The listing builds one solid part. Answer for the finished solid, in the listing's coordinates (mm). Face numbers are marked on the shaded views. A direction names the side the tool comes from. Give positions to 0.01 mm unless a question says otherwise; leave off trailing zeros. Order: outer loops, then holes, each group sorted by start corner. A loop starts at its lowest first (then second) coordinate and runs counter-clockwise, first axis right, second up. Notation, with made-up numbers: (-15, -8) - (4, -8) arc R27 cw to (4, 20) - close; hole circle Ø1 at (9, 21.5). An arc over 180 degrees is marked (long way). Answer as a JSON object with one key per item and string values. Group by question number.
Q1. The mould has two halves that part along X. Classify the marked faces 3, 4, 5 and 6: released by +X, released by -X, zero draft, split by the parting line, or undercut.
Q2. Given pin 1 (5 mm diameter, centred on y = 6.5, z = -6, fed in from +X); pin 2 (3.5 mm diameter, centred on x = -2, y = 10, fed in from -Z); pin 3 (1 mm diameter, centred on y = -6, z = -4, fed in from +X), each flat-ended and moving along its own axis, determine where each tip first touches the part or whether it passes through.
Q3. For the marked faces 1 and 2, determine the directions among +Z, -Z, +X, -X, +Y, -Y from which every point of the face is accessible in a straight line to the end or side of a thin tool.
Q4. A cutting plane is placed at D-D, the plane z = -6.75. Give the vertices of the cut face in (x, y), and give its area (3 significant figures).
Q5. A cutting plane is placed at B-B, the plane z = -1. Give the vertices of the cut face in (x, y), and give its area (3 significant figures).
Q6. A cutting plane is placed at A-A, the plane x = 0. Give the vertices of the cut face in (y, z), and give its area (3 significant figures).
Q7. A cutting plane is placed at C-C, the plane y = -17. Give the vertices of the cut face in (x, z), and give its area (3 significant figures).
Q8. Consider line 1 (Y direction, x = 0, z = -2.85); line 2 (Y direction, x = 0, z = -1.15); line 3 (Y direction, x = 0, z = -7.9). Determine where each line is inside the solid, lowest interval first.
from build123d import *

# Parameters (mm, degrees)
BOSS_EXTRUDE1_DEPTH = 4
SKETCH5_R           = 6
BOSS_EXTRUDE3_DEPTH = 6
SKETCH6_R           = 3
CUT_EXTRUDE1_DEPTH  = 5
SKETCH7_R           = 1.5
CUT_EXTRUDE2_DEPTH  = 6
SKETCH4_R           = 1.6
CUT_EXTRUDE3_DEPTH  = 11
SKETCH8_R           = 3
CUT_EXTRUDE4_DEPTH  = 1.5


with BuildPart() as part:
    # Sketch1 → Boss-Extrude1 (new body)
    with BuildSketch(Plane.XY):
        with BuildLine():
            Line((3, 17.5), (5.908426238, 1.044269788))
            ThreePointArc((5.908426238, 1.044269788), (6, 0), (5.908426238, -1.044269788))
            Line((5.908426238, -1.044269788), (3, -17.5))
            ThreePointArc((3, -17.5), (0, -20.5), (-3, -17.5))
            Line((-3, -17.5), (-5.908426238, -1.044269788))
            ThreePointArc((-5.908426238, -1.044269788), (-6, 0), (-5.908426238, 1.044269788))
            Line((-5.908426238, 1.044269788), (-3, 17.5))
            ThreePointArc((-3, 17.5), (0, 20.5), (3, 17.5))
        make_face()
    extrude(amount=-BOSS_EXTRUDE1_DEPTH)

    # Sketch5 → Boss-Extrude3 (add)
    with BuildSketch(Plane(origin=(0, 0, -4), x_dir=(-1, 0, 0), z_dir=(0, 0, -1))):
        Circle(SKETCH5_R)
    extrude(amount=BOSS_EXTRUDE3_DEPTH)

    # Sketch6 → Cut-Extrude1 (cut)
    with BuildSketch(Plane(origin=(0, 0, -10), x_dir=(-1, 0, 0), z_dir=(0, 0, -1))):
        Circle(SKETCH6_R)
    extrude(amount=-CUT_EXTRUDE1_DEPTH, mode=Mode.SUBTRACT)

    # Sketch7 → Cut-Extrude2 (cut, through all)
    with BuildSketch(Plane(origin=(0, 0, -5), x_dir=(-1, 0, 0), z_dir=(0, 0, -1))):
        Circle(SKETCH7_R)
    extrude(amount=-CUT_EXTRUDE2_DEPTH, mode=Mode.SUBTRACT)

    # Sketch4 → Cut-Extrude3 (cut, through all)
    with BuildSketch(Plane.XY):
        with Locations((0, 17.5)):
            Circle(SKETCH4_R)
        with Locations((0, -17.5)):
            Circle(SKETCH4_R)
    extrude(amount=-CUT_EXTRUDE3_DEPTH, mode=Mode.SUBTRACT)

    # Sketch8 → Cut-Extrude4 (cut)
    with BuildSketch(Plane.XY):
        Circle(SKETCH8_R)
    extrude(amount=-CUT_EXTRUDE4_DEPTH, mode=Mode.SUBTRACT)


solid = part.part
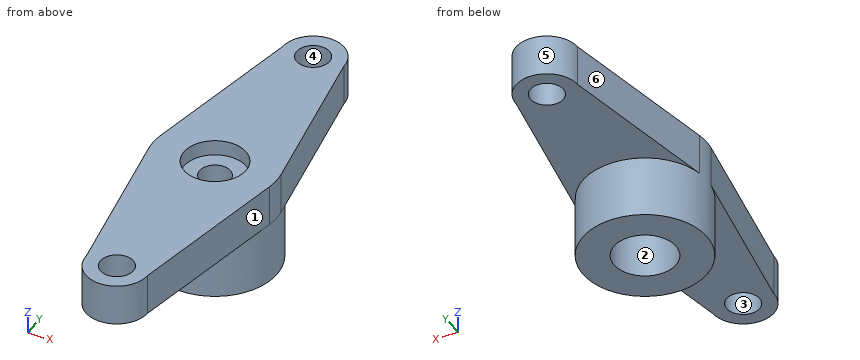
Reply:
{
 "1": {"face 3": "undercut", "face 4": "undercut", "face 5": "split by the parting line", "face 6": "released by -X"},
 "2": {"pin 1": "stops at x = 5.21", "pin 2": "stops at z = -4", "pin 3": "stops at x = 5.12"},
 "3": {"face 1": "+Z, -Z, +X, -Y", "face 2": "-Z"},
 "4": {"outline": "circle Ø12 at (0, 0); hole circle Ø6 at (0, 0)", "area": "84.8 mm^2"},
 "5": {"outline": "(-5.91, -1.04) - (-3, -17.5) arc R3 ccw to (3, -17.5) - (5.91, -1.04) arc R6 ccw to (5.91, 1.04) - (3, 17.5) arc R3 ccw to (-3, 17.5) - (-5.91, 1.04) arc R6 ccw to start; hole circle Ø6 at (0, 0); hole circle Ø3.2 at (0, -17.5); hole circle Ø3.2 at (0, 17.5)", "area": "302 mm^2"},
 "6": {"outline": "(-20.5, -4) - (-19.1, -4) - (-19.1, 0) - (-20.5, 0) - close; (-15.9, -4) - (-6, -4) - (-6, -10) - (-3, -10) - (-3, -5) - (-1.5, -5) - (-1.5, -1.5) - (-3, -1.5) - (-3, 0) - (-15.9, 0) - close; (1.5, -5) - (3, -5) - (3, -10) - (6, -10) - (6, -4) - (15.9, -4) - (15.9, 0) - (3, 0) - (3, -1.5) - (1.5, -1.5) - close; (19.1, -4) - (20.5, -4) - (20.5, 0) - (19.1, 0) - close", "area": "161 mm^2"},
 "7": {"outline": "(-3.09, -4) - (-1.52, -4) - (-1.52, 0) - (-3.09, 0) - close; (1.52, -4) - (3.09, -4) - (3.09, 0) - (1.52, 0) - close", "area": "12.5 mm^2"},
 "8": {"line 1": "y = -20.5 to -19.1, -15.9 to -1.5, 1.5 to 15.9, 19.1 to 20.5", "line 2": "y = -20.5 to -19.1, -15.9 to -3, 3 to 15.9, 19.1 to 20.5", "line 3": "y = -6 to -3, 3 to 6"}
}
